Here's how the part is built. I have some questions about the finished solid (model axes, mm). A direction names the side the tool comes from. Give positions to 0.01 mm unless a question says otherwise; leave off trailing zeros. Loops run counter-clockwise (first coordinate to the right, second up) from the corner with the lowest first, then second, coordinate; pieces in that order, holes last. Notation, with made-up numbers: (29, 74) - (51, 74) arc R31 ccw to (51, 113) - close; hole circle Ø4 at (-38, 52.5). An arc over 180 degrees is marked (long way). Use one line per item in the form item = value.
from build123d import *

# Parameters (mm, degrees)
F0_W     = 684.5037638012
F0_H     = 19.05
F0_W_2   = 1162.05
F0_W_3   = 19.05
F0_H_2   = 217.7895105028
F0_H_3   = 38.1
F0_W_4   = 9.525
F1_DEPTH = 19.05
F2_DEPTH = 241.3
F3_DEPTH = 38.1


with BuildPart() as f1:
    # F0 (on Top) → F1 (new body)
    with BuildSketch(Plane.XY):
        Polygon((-205.0596728024, 4.7625), (205.0596728024, 4.7625), (609.6, 104.4729894972), (590.55, 104.4729894972), (590.55, 322.2625), (571.5, 322.2625), (571.5, 341.3125), (581.025, 341.3125), (581.025, 360.3625), (-581.025, 360.3625), (-581.025, 341.3125), (-571.5, 341.3125), (-571.5, 322.2625), (-590.55, 322.2625), (-590.55, 104.4729894972), (-609.6, 104.4729894972), align=None)
        Polygon((-586.3576715827, 123.2287481447), (-48.5401919344, 76.1273604725), (-50.202205622, 57.15), (-588.0196852703, 104.2513876722), align=None, mode=Mode.SUBTRACT)
        Polygon((-19.05, 57.15), (-19.05, 76.2), (-9.525, 76.2), (-9.525, 114.3), (9.525, 114.3), (9.525, 76.2), (19.05, 76.2), (19.05, 57.15), align=None, mode=Mode.SUBTRACT)
        Polygon((588.0196852703, 104.2513876722), (50.202205622, 57.15), (48.5401919344, 76.1273604725), (586.3576715827, 123.2287481447), align=None, mode=Mode.SUBTRACT)
        Polygon((-17.4948285758, 85.9344063425), (-25.2456829409, 68.5324881549), (-573.0551714242, 312.5280936575), (-565.3043170591, 329.9300118451), align=None, mode=Mode.SUBTRACT)
        Polygon((25.2456829409, 68.5324881549), (17.4948285758, 85.9344063425), (565.3043170591, 329.9300118451), (573.0551714242, 312.5280936575), align=None, mode=Mode.SUBTRACT)
        with Locations((0, 242.8875)):
            Rectangle(F0_W, F0_H, mode=Mode.SUBTRACT)
        with Locations((0, 369.8875)):
            Rectangle(F0_W_2, F0_H)
        with Locations((0, 242.8875)):
            Rectangle(F0_W, F0_H)
        Polygon((565.3043170591, 329.9300118451), (17.4948285758, 85.9344063425), (25.2456829409, 68.5324881549), (573.0551714242, 312.5280936575), align=None)
        Polygon((-573.0551714242, 312.5280936575), (-25.2456829409, 68.5324881549), (-17.4948285758, 85.9344063425), (-565.3043170591, 329.9300118451), align=None)
        Polygon((-50.202205622, 57.15), (-48.5401919344, 76.1273604725), (-586.3576715827, 123.2287481447), (-588.0196852703, 104.2513876722), align=None)
        Polygon((48.5401919344, 76.1273604725), (50.202205622, 57.15), (588.0196852703, 104.2513876722), (586.3576715827, 123.2287481447), align=None)
        with Locations((-600.075, 213.3677447486)):
            Rectangle(F0_W_3, F0_H_2)
        with Locations((600.075, 213.3677447486)):
            Rectangle(F0_W_3, F0_H_2)
        Polygon((590.55, 322.2625), (609.6, 322.2625), (609.6, 341.3125), (600.075, 341.3125), (581.025, 341.3125), (571.5, 341.3125), (571.5, 322.2625), align=None)
        Polygon((-9.525, 76.2), (-19.05, 76.2), (-19.05, 57.15), (19.05, 57.15), (19.05, 76.2), (9.525, 76.2), align=None)
        Polygon((-609.6, 341.3125), (-609.6, 322.2625), (-590.55, 322.2625), (-571.5, 322.2625), (-571.5, 341.3125), (-581.025, 341.3125), (-600.075, 341.3125), align=None)
        Polygon((-600.075, 379.4125), (-600.075, 341.3125), (-581.025, 341.3125), (-581.025, 360.3625), (-581.025, 379.4125), align=None)
        with Locations((0, 95.25)):
            Rectangle(F0_W_3, F0_H_3)
        Polygon((581.025, 341.3125), (600.075, 341.3125), (600.075, 379.4125), (581.025, 379.4125), (581.025, 360.3625), align=None)
        with Locations((-604.8375, 360.3625)):
            Rectangle(F0_W_4, F0_H_3)
        with Locations((604.8375, 360.3625)):
            Rectangle(F0_W_4, F0_H_3)
    extrude(amount=F1_DEPTH)

    # F0 (on Top) → F2 (join)
    with BuildSketch(Plane.XY):
        Polygon((-609.6, 341.3125), (-609.6, 322.2625), (-590.55, 322.2625), (-571.5, 322.2625), (-571.5, 341.3125), (-581.025, 341.3125), (-600.075, 341.3125), align=None)
        Polygon((-9.525, 76.2), (-19.05, 76.2), (-19.05, 57.15), (19.05, 57.15), (19.05, 76.2), (9.525, 76.2), align=None)
        Polygon((590.55, 322.2625), (609.6, 322.2625), (609.6, 341.3125), (600.075, 341.3125), (581.025, 341.3125), (571.5, 341.3125), (571.5, 322.2625), align=None)
        Polygon((581.025, 341.3125), (600.075, 341.3125), (600.075, 379.4125), (581.025, 379.4125), (581.025, 360.3625), align=None)
        with Locations((0, 95.25)):
            Rectangle(F0_W_3, F0_H_3)
        Polygon((-600.075, 379.4125), (-600.075, 341.3125), (-581.025, 341.3125), (-581.025, 360.3625), (-581.025, 379.4125), align=None)
    extrude(amount=-F2_DEPTH)

    # F0 (on Top) → F3 (join)
    with BuildSketch(Plane.XY):
        with Locations((-600.075, 213.3677447486)):
            Rectangle(F0_W_3, F0_H_2)
        Polygon((-50.202205622, 57.15), (-48.5401919344, 76.1273604725), (-586.3576715827, 123.2287481447), (-588.0196852703, 104.2513876722), align=None)
        Polygon((-573.0551714242, 312.5280936575), (-25.2456829409, 68.5324881549), (-17.4948285758, 85.9344063425), (-565.3043170591, 329.9300118451), align=None)
        with Locations((0, 369.8875)):
            Rectangle(F0_W_2, F0_H)
        Polygon((565.3043170591, 329.9300118451), (17.4948285758, 85.9344063425), (25.2456829409, 68.5324881549), (573.0551714242, 312.5280936575), align=None)
        with Locations((600.075, 213.3677447486)):
            Rectangle(F0_W_3, F0_H_2)
        Polygon((48.5401919344, 76.1273604725), (50.202205622, 57.15), (588.0196852703, 104.2513876722), (586.3576715827, 123.2287481447), align=None)
        with Locations((0, 242.8875)):
            Rectangle(F0_W, F0_H)
    extrude(amount=-F3_DEPTH)


solid = f1.part
(1) If we section it at C-C (x = -370): List the corners of the cut face in (y, z) for me.
Geometry says:
outline = (45.42, 0) - (85.16, 0) - (85.16, -38.1) - (104.28, -38.1) - (104.28, 0) - (222.09, 0) - (222.09, -38.1) - (242.94, -38.1) - (242.94, 0) - (360.36, 0) - (360.36, -38.1) - (379.41, -38.1) - (379.41, 19.05) - (45.42, 19.05) - close
(2) If we section it at B-B (y = 282): List the corners of the cut face in (x, z) for me.
Geometry says:
outline = (-609.6, -38.1) - (-590.55, -38.1) - (-590.55, 0) - (-504.51, 0) - (-504.51, -38.1) - (-457.69, -38.1) - (-457.69, 0) - (457.69, 0) - (457.69, -38.1) - (504.51, -38.1) - (504.51, 0) - (590.55, 0) - (590.55, -38.1) - (609.6, -38.1) - (609.6, 19.05) - (-609.6, 19.05) - close
(3) If we section it at A-A (z = -152.5): Give the number of separate pieces and of enclosed holes in the cut face, plus the area to 3 significant figures.
Geometry says:
separate_pieces = 3
enclosed_holes = 0
area = 4,350 mm²
(4) If I drill on probe 1 along Y at (x, z) = (379, -26.5); probe 2 along X at (y, z) = (337, -73.5); probe 3 along Y at (x, z) = (-10.5, -29), over which ranges is the centre line in solid material (lowest first)?
Geometry says:
probe_1 = 85.95 to 105.07, 226.1 to 246.95, 360.36 to 379.41
probe_2 = -609.6 to -571.5, 571.5 to 609.6
probe_3 = 57.15 to 76.2, 233.36 to 252.41, 360.36 to 379.41
(5) Thinking about a two-plate mould opening in Y: for faces 6 (the flat face through (-8, 360.362, -19)), 7 (the flat face through (404.5, 53.92, 9.39)), 8 (the flat face through (317, 90, -38.1)), which applies, pulls with the +Y half, pulls with the -Y half, needs draft (parallel to the pull), parting line crosses it, or undercut?
Geometry says:
face_6 = undercut
face_7 = pulls with the -Y half
face_8 = needs draft
(6) For faces 1 (the flat face through (590, 345, -241.3)), 2 (the flat face through (-5, 233.362, -19)), 3 (the flat face through (590.55, 212, -19)), 4 (the flat face through (315.35, 80.37, -18.78)), 5 (the flat face through (-600.075, 361, -119)), which set-ups out of +Z, -Z, +X, -X, +Y, -Y let a thin tool reach every point of the face, with its end or its side?
Geometry says:
face_1 = -Z, +X, -X, +Y, -Y
face_2 = -Z
face_3 = -Z, -Y
face_4 = -Z, +X, -Y
face_5 = -Z, -X, +Y
(7) For P1, Ø12, axis at x = 250.5, y = 127.5, coming from the -Z side; P2, Ø9.5, axis at x = -598.5, z = -18, coming from the -Y side; P3, Ø9.5, axis at x = 36, y = 242.5, coming from the -Z side, each with a flat end and sliding along its axis, tell me the tip position at first contact or that it passes through.
Geometry says:
P1 = 0
P2 = 104.47
P3 = -38.1
